Could you check a few things on this drawing? It's one solid part, dimensions in mm from its lowest x, y, z. A direction names the side the tool comes from. Round coordinates to 2 decimals unless told otherwise and drop trailing zeros. Write each loop counter-clockwise with the first axis right and the second up, starting at its lowest first coordinate (ties: lowest second). Pieces come first, ordered by that corner, then holes. Notation, with made-up numbers: (75, -9.5) -> (105, -9.5) arc R7 cw to (105, 0.5) -> close; hole circle Ø2 at (41, 23.5). An arc over 180 degrees is marked (long way). Answer in a Markdown table with one row per item. Add a question column.
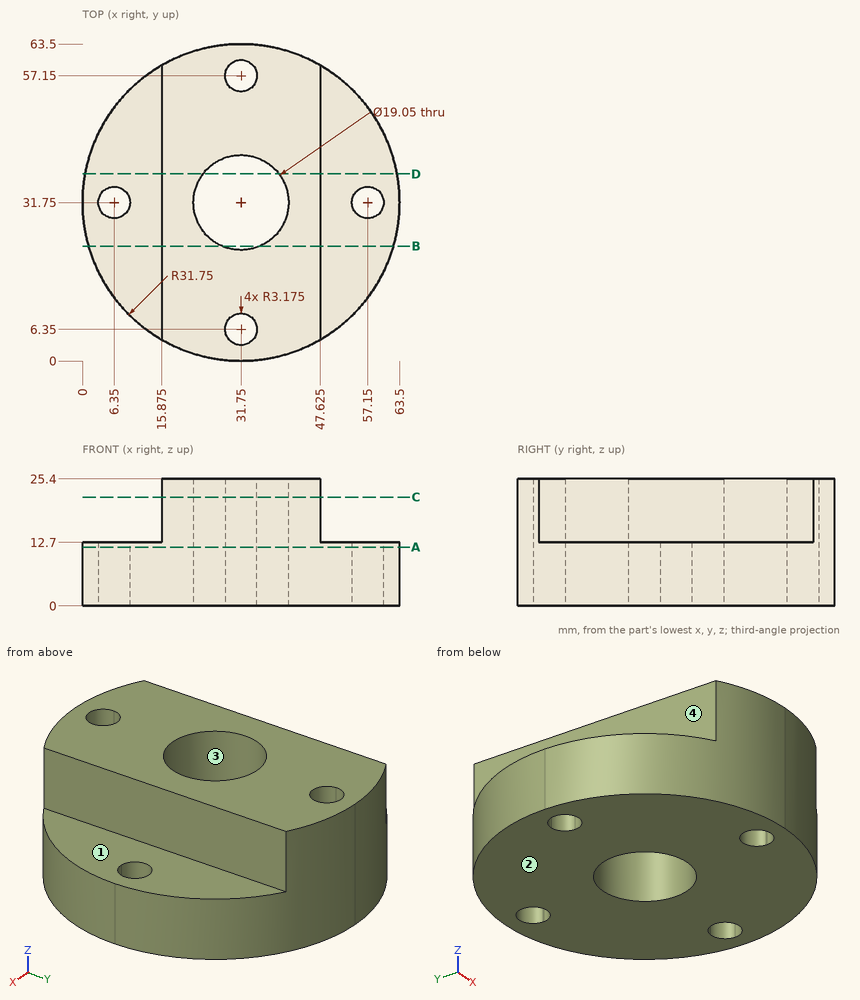
(1) Suppose I cut it at A-A, the plane z = 11.75. Please give me the cut outline in (x, y) (3 decimals).
(2) If we mould it in two halves opening along Y, with no side actions, what happens to the marked faces 3 and 4? For each: pulls with the +Y half, pulls with the -Y half, needs draft (parallel to the pull), parting line crosses it, or undercut.
(3) Suppose I cut it at C-C, the plane z = 21.75. Please give me the cut outline in (x, y) (3 decimals), then the cut area to 3 significant figures.
(4) Suppose I cut it at D-D, the plane y = 37.5. Please give me the cut outline in (x, z) (3 decimals), then the cut area to 3 significant figures.
(5) I need wall thicknesses on L1, parallel to X at y = 31.75, z = 11.5 (3 decimals); L2, parallel to X at y = 31.75, z = 12.75 (3 decimals); L3, parallel to Y at x = 31, z = 20. Which ranges of each line are inside material? Lowest first, please.
(6) For P1, Ø1.5, axis at x = 51.5, y = 16, coming from the +Z side; P2, Ø10, axis at x = 21.5, z = 18, coming from the +Y side; P3, Ø4, axis at y = 28, z = 20, coming from the -X side (3 decimals); P4, Ø11.5, axis at x = 31.75, y = 31.75, coming from the +Z side, each with a flat end and sliding along its axis, tell me the tip position at first contact or that it passes through.
(7) Suppose I cut it at B-B, the plane y = 23. Please give me the cut outline in (x, z) (3 decimals).
(8) On a 3-axis mill with a long thin cutter (end or side, diameter ignored), from which of +Z, -Z, +X, -X, +Y, -Y can I reach the whole of each face in a straight line? I mean the marked faces 1 and 2. Say none if no direction works.
Response:
| question | item | result |
|---|---|---|
| 1 | outline | circle Ø63.5 at (31.75, 31.75); hole circle Ø6.35 at (6.35, 31.75); hole circle Ø19.05 at (31.75, 31.75); hole circle Ø6.35 at (31.75, 6.35); hole circle Ø6.35 at (31.75, 57.15); hole circle Ø6.35 at (57.15, 31.75) |
| 2 | face 3 | undercut |
| 2 | face 4 | needs draft |
| 3 | outline | (15.875, 4.254) arc R31.75 ccw to (47.625, 4.254) -> (47.625, 59.246) arc R31.75 ccw to (15.875, 59.246) -> close; hole circle Ø19.05 at (31.75, 31.75); hole circle Ø6.35 at (31.75, 6.35); hole circle Ø6.35 at (31.75, 57.15) |
| 3 | area | 1,580 mm² |
| 4 | outline | (0.525, 0) -> (24.156, 0) -> (24.156, 25.4) -> (15.875, 25.4) -> (15.875, 12.7) -> (0.525, 12.7) -> close; (39.344, 0) -> (62.975, 0) -> (62.975, 12.7) -> (47.625, 12.7) -> (47.625, 25.4) -> (39.344, 25.4) -> close |
| 4 | area | 811 mm² |
| 5 | L1 | 0 to 3.175, 9.525 to 22.225, 41.275 to 53.975, 60.325 to 63.5 |
| 5 | L2 | 15.875 to 22.225, 41.275 to 47.625 |
| 5 | L3 | 0.01 to 3.26, 9.44 to 22.25, 41.25 to 54.06, 60.24 to 63.49 |
| 6 | P1 | z = 12.7 |
| 6 | P2 | y = 63.06 |
| 6 | P3 | x = 15.875 |
| 6 | P4 | through |
| 7 | outline | (1.23, 0) -> (27.987, 0) -> (27.987, 25.4) -> (15.875, 25.4) -> (15.875, 12.7) -> (1.23, 12.7) -> close; (35.513, 0) -> (62.27, 0) -> (62.27, 12.7) -> (47.625, 12.7) -> (47.625, 25.4) -> (35.513, 25.4) -> close |
| 8 | face 1 | +Z, +X, +Y, -Y |
| 8 | face 2 | -Z, +X, -X, +Y, -Y |
